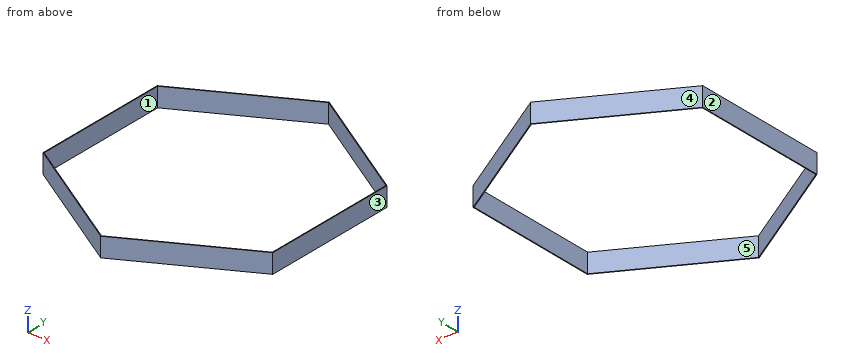
Autodesk Inventor part; units mm, degrees
ref_plane "Work Plane1" through (0, 0, 0) normal (0, 0, 1) x (1, 0, 0)
ref_plane "YZ Plane" through (0, 0, 0) normal (1, 0, 0) x (0, 1, 0)
ref_plane "XZ Plane" through (0, 0, 0) normal (0, 1, 0) x (-1, 0, 0)
ref_plane "Work Plane1" through (0, 0, 0) normal (0, 0, 1) x (1, 0, 0)
sketch "Sketch1" plane through (0, 0, 0) normal (0, 0, 1) x (1, 0, 0)
  line L0 (300, -173.2051) -> (0, -346.4102)
  line L1 (0, -346.4102) -> (-300, -173.2051)
  line L2 (-300, -173.2051) -> (-300, 173.2051)
  line L3 (-300, 173.2051) -> (0, 346.4102)
  line L4 (0, 346.4102) -> (300, 173.2051)
  line L5 (300, 173.2051) -> (300, -173.2051)
  line L6 (302, 174.3598) -> (302, -174.3598)
  line L7 (302, -174.3598) -> (0, -348.7196)
  line L8 (0, -348.7196) -> (-302, -174.3598)
  line L9 (-302, -174.3598) -> (-302, 174.3598)
  line L10 (-302, 174.3598) -> (0, 348.7196)
  line L11 (0, 348.7196) -> (302, 174.3598)
  point P0 (0, 0)
  point P1 (0, 0)
  point P2 (0, 0)
  dimension "d0" = 302
  dimension "d1" = 300
extrude "Extrusion1" add sketch "Sketch1" along normal blind 50
properties part number "Wallmesh"
CAD build for the part. Positions are in the model's coordinates, mm. Face numbers are marked on the shaded views. A direction names the side the tool comes from. Coordinates: 2 decimals unless noted, no trailing zeros. Loops run counter-clockwise (first coordinate to the right, second up) from the corner with the lowest first, then second, coordinate; pieces in that order, holes last. Notation, with made-up numbers: (88.5, -39) - (94.5, -39) arc R11 cw to (94.5, -31) - close; hole circle Ø6 at (-5.5, 55.5). An arc over 180 degrees is marked (long way). Return JSON: item names as keys, results as strings.
1. Mould opens along X. For the marked faces 3, 4 and 5 say: released by +X, released by -X, zero draft, split by the parting line, or undercut.
Result:
{"face 3": "released by +X", "face 4": "released by -X", "face 5": "undercut"}
2. Band-saw the part on A-A (y = -77.5). Give the cut face in (x, z), and give its area (3 significant figures).
Result:
{"outline": "(-302, 0) - (-300, 0) - (-300, 50) - (-302, 50) - close; (300, 0) - (302, 0) - (302, 50) - (300, 50) - close", "area": "200 mm2"}
3. Band-saw the part on C-C (x = 167). Give the cut face in (y, z).
Result:
{"outline": "(-252.3, 0) - (-249.99, 0) - (-249.99, 50) - (-252.3, 50) - close; (249.99, 0) - (252.3, 0) - (252.3, 50) - (249.99, 50) - close"}
4. 3-axis set-ups, long thin cutter, end or side, ignore diameter. For the marked faces 1 and 2: which of +Z, -Z, +X, -X, +Y, -Y reach the whole face in a straight line?
Result:
{"face 1": "+Z, -Z", "face 2": "+Z, -Z, -X, +Y, -Y"}
5. Probe L1, parallel to X at y = -169.5, z = 14; L2, parallel to X at y = -234, z = 5.5; L3, parallel to Y at x = -268.5, z = 5. List the from-to ranges inside material, lowest first. Write a range as from..to.
Result:
{"L1": "x = -302..-300, 300..302", "L2": "x = -198.7..-194.7, 194.7..198.7", "L3": "y = -193.7..-191.39, 191.39..193.7"}
6. Drop flat-ended pins along their axis: pin 1 (2 mm diameter, centred on x = 144.5, z = 34, fed in from +Y); pin 2 (10 mm diameter, centred on x = 236.5, z = 43.5, fed in from +Y); pin 3 (1.5 mm diameter, centred on y = 244, z = 28, fed in from +X). Give the stop position or say it passes through.
Result:
{"pin 1": "stops at y = 265.87", "pin 2": "stops at y = 215.06", "pin 3": "stops at x = 182.68"}
7. Band-saw the part on B-B (z = 38). Give the cut face in (x, y).
Result:
{"outline": "(-302, -174.36) - (0, -348.72) - (302, -174.36) - (302, 174.36) - (0, 348.72) - (-302, 174.36) - close; hole (-300, -173.21) - (0, -346.41) - (300, -173.21) - (300, 173.21) - (0, 346.41) - (-300, 173.21) - close"}
